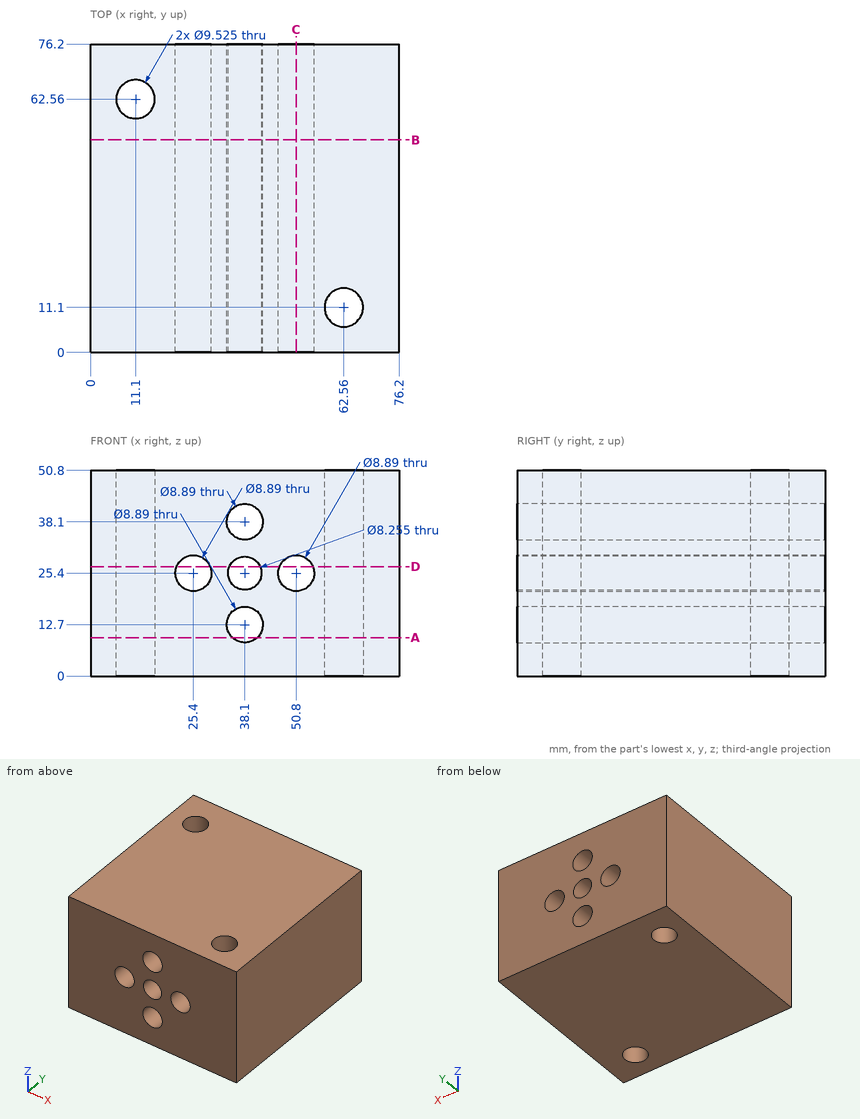
Drawing for the job (mm, zero at the part's lowest x, y, z). Give positions to 0.01 mm unless a question says otherwise; leave off trailing zeros. Order: outer loops, then holes, each group sorted by start corner. A loop starts at its lowest first (then second) coordinate and runs counter-clockwise, first axis right, second up. Notation, with made-up numbers: (7, 56) - (14, 56) arc R5 ccw to (14, 62) - close; hole circle Ø1 at (18, 62). An arc over 180 degrees is marked (long way). Write item = value, one per line. Start each with the question number.
1. Cut at C-C, the plane x = 50.8. List the corners of the cut face in (y, z) (3 decimals), and give its area (3 significant figures).
2. Cut at D-D, the plane z = 27. List the corners of the cut face in (x, y) (1 decimal).
3. Cut at B-B, the plane y = 52.5. List the corners of the cut face in (x, z) (1 decimal), and give its area (3 significant figures).
4. Cut at A-A, the plane z = 9.5. List the corners of the cut face in (x, y) (1 decimal).
5. Probe line 1 along Z through (x, y) = (38, 41); line 2 along X through (y, z) = (33, 25.4) (1 decimal); line 3 along X through (y, z) = (22.5, 12.5). List the from-to ranges inside material, lowest first.
Taken from the geometry:
q1.outline = (0, 0) - (76.2, 0) - (76.2, 20.955) - (0, 20.955) - close; (0, 29.845) - (76.2, 29.845) - (76.2, 50.8) - (0, 50.8) - close
q1.area = 3,190 mm²
q2.outline = (0, 0) - (21.3, 0) - (21.3, 76.2) - (0, 76.2) - close; (29.5, 0) - (34.3, 0) - (34.3, 76.2) - (29.5, 76.2) - close; (41.9, 0) - (46.7, 0) - (46.7, 76.2) - (41.9, 76.2) - close; (54.9, 0) - (76.2, 0) - (76.2, 76.2) - (54.9, 76.2) - close; hole circle Ø9.5 at (11.1, 62.6); hole circle Ø9.5 at (62.6, 11.1)
q3.outline = (0, 0) - (76.2, 0) - (76.2, 50.8) - (0, 50.8) - close; hole circle Ø8.9 at (25.4, 25.4); hole circle Ø8.9 at (38.1, 12.7); hole circle Ø8.9 at (38.1, 38.1); hole circle Ø8.3 at (38.1, 25.4); hole circle Ø8.9 at (50.8, 25.4)
q3.area = 3,570 mm²
q4.outline = (0, 0) - (35, 0) - (35, 76.2) - (0, 76.2) - close; (41.2, 0) - (76.2, 0) - (76.2, 76.2) - (41.2, 76.2) - close; hole circle Ø9.5 at (11.1, 62.6); hole circle Ø9.5 at (62.6, 11.1)
q5.line_1 = 0 to 8.26, 17.14 to 21.27, 29.53 to 33.66, 42.54 to 50.8
q5.line_2 = 0 to 21, 29.8 to 34, 42.2 to 46.4, 55.2 to 76.2
q5.line_3 = 0 to 33.66, 42.54 to 76.2
